from build123d import *

# Parameters (mm, degrees)
SKETCH1_R               = 44.137005248
BOSS_EXTRUDE1_DEPTH     = 2.54
SKETCH2_W               = 7.363975328
SKETCH2_H               = 35.413609254
CUT_EXTRUDE1_DEPTH      = 2.54
BOSS_EXTRUDE2_START     = -6.36773
BOSS_EXTRUDE2_DEPTH     = 35.413609254
CIRPATTERN3_COUNT       = 4
SKETCH6_R               = 46.929171811
SKETCH6_R_2             = 44.137005248
BOSS_EXTRUDE3_DEPTH     = 54.102
CUT_EXTRUDE2_DEPTH      = 86.62546781
CUT_EXTRUDE2_DEPTH_BACK = 86.62546781


with BuildPart() as part:
    # Sketch1 → Boss-Extrude1 (new body)
    with BuildSketch(Plane(origin=(0, 0, 0), x_dir=(1, 0, 0), z_dir=(0, 1, 0))):
        with Locations(Location((0, 0, 0), (0, 0, 270))):
            Circle(SKETCH1_R)
    extrude(amount=BOSS_EXTRUDE1_DEPTH)

    # Sketch2 → Cut-Extrude1 (cut)
    with BuildSketch(Plane(origin=(0, 2.54, 0), x_dir=(1, 0, 0), z_dir=(0, 1, 0))):
        with Locations((0, 24.074534725)):
            Rectangle(SKETCH2_W, SKETCH2_H)
    cut_extrude1 = extrude(amount=-CUT_EXTRUDE1_DEPTH, mode=Mode.SUBTRACT)

    # Sketch3 → Boss-Extrude2 (add)
    with BuildSketch(Plane.XY.offset(BOSS_EXTRUDE2_START)):
        Polygon((3.681987664, 2.54), (-3.464612865, 7.544103563), (2.37831785, 7.544103563), (9.524918378, 2.54), align=None)
    boss_extrude2 = extrude(amount=-BOSS_EXTRUDE2_DEPTH)

    # CirPattern3: Cut-Extrude1, Boss-Extrude2 ×4 about axis
    cirpattern3_axis = Axis((0, 0, 0), (0, 1, 0))
    add([cut_extrude1.rotate(cirpattern3_axis, i * 360 / CIRPATTERN3_COUNT) for i in range(1, CIRPATTERN3_COUNT)], mode=Mode.SUBTRACT)
    add([boss_extrude2.rotate(cirpattern3_axis, i * 360 / CIRPATTERN3_COUNT) for i in range(1, CIRPATTERN3_COUNT)])

    # Sketch6 → Boss-Extrude3 (add)
    with BuildSketch(Plane(origin=(0, 0, 0), x_dir=(1, 0, 0), z_dir=(0, 1, 0))):
        with Locations(Location((0, 0, 0), (0, 0, 270))):
            Circle(SKETCH6_R)
        with Locations(Location((0, 0, 0), (0, 0, 270))):
            Circle(SKETCH6_R_2, mode=Mode.SUBTRACT)
    extrude(amount=BOSS_EXTRUDE3_DEPTH)

    # Sketch7 → Cut-Extrude2 (cut, two sides: drawn at the far end of the back side and taken through both)
    with BuildSketch(Plane(origin=(0, 0, 0), x_dir=(0, 0, -1), z_dir=(1, 0, 0)).offset(-CUT_EXTRUDE2_DEPTH_BACK)):
        Polygon((0, 54.102), (-46.929171811, 5.913652035), (-46.929171811, 54.102), align=None)
    extrude(amount=CUT_EXTRUDE2_DEPTH + CUT_EXTRUDE2_DEPTH_BACK, mode=Mode.SUBTRACT)


solid = part.part
Design review of the part built by this model. Coordinates are the model's own, in mm. A direction names the side the tool comes from. Round coordinates to 2 decimals unless told otherwise and drop trailing zeros. Write each loop counter-clockwise with the first axis right and the second up, starting at its lowest first coordinate (ties: lowest second). Pieces come first, ordered by that corner, then holes. Notation, with made-up numbers: (53.25, 33) -> (110.25, 33) arc R37 ccw to (110.25, 72) -> close; hole circle Ø10 at (44.25, 32). An arc over 180 degrees is marked (long way). One line per item, written item: value. Start each with the question number.
Q1. Add section D-D (y = 49.5). Give the boundary of the cut face in (x, z).
Q2. To check wall thickness, follow probe 1 along X at (y, z) = (40, 0); probe 2 along Y at (x, z) = (-32, -28); probe 3 along X at (y, z) = (27.5, 21). State the ranges of each line that lie inside material, in increasing order.
Q3. Add section C-C (x = 0). Give the boundary of the cut face in (y, z), then the cut area to 3 significant figures.
Q4. Tool access review of faces 1 (the face through (-41.781, 5, -3)), 2 (the face through (0.2, 54.102, -44.4)), 3 (the face through (-0.159, 5.007, 23.827)), 4 (the face through (24, 1, -3.682)): name each direction out of +Z, -Z, +X, -X, +Y, -Y from which nothing blocks a thin tool from reaching the whole face with its end or side.
Q5. The part is to be moulded in two halves that separate along X. For faces 5 (the face through (2.063, 20.661, -46.884)), 6 (the face through (6.368, 5, 3)), 7 (the face through (3.257, 8.703, 44.212)), 8 (the face through (-3.682, 1, 24)), say which applies: pulls with the +X half, pulls with the -X half, needs draft (parallel to the pull), parting line crosses it, or undercut.
Q6. Add section A-A (z = -16.5). Give the boundary of the cut face in (x, y), then the cut area to 3 significant figures.
Q7. Add section B-B (x = 27.5). Give the boundary of the cut face in (y, z), then the cut area to 3 significant figures.
Q8. Insertion check: P1, Ø0.8, axis at x = -1.5, y = 1, coming from the -Z side; P2, Ø3, axis at y = 16, z = -28.5, coming from the -X side; P3, Ø12, axis at y = 46, z = -10, coming from the +X side. Each pin has a flat end and moves straight along its axis. Give the tip position at first contact, or say it passes through.
Response:
1. outline: (-46.71, 4.48) arc R46.93 ccw (long way) to (46.71, 4.48) -> (43.91, 4.48) arc R44.14 cw (long way) to (-43.91, 4.48) -> close
2. probe 1: x = -46.93 to -44.14, 44.14 to 46.93
2. probe 2: y = 0 to 2.54
2. probe 3: x = -41.97 to -38.82, 38.82 to 41.97
3. outline: (0, -46.93) -> (54.1, -46.93) -> (54.1, -44.14) -> (2.54, -44.14) -> (2.54, -41.78) -> (0, -41.78) -> close; (0, -6.37) -> (2.54, -6.37) -> (2.54, 6.37) -> (0, 6.37) -> close; (0, 41.78) -> (2.54, 41.78) -> (2.54, 44.14) -> (8.78, 44.14) -> (5.91, 46.93) -> (0, 46.93) -> close; (5.12, -41.78) -> (7.54, -41.78) -> (7.54, -6.37) -> (5.12, -6.37) -> close; (5.12, 6.37) -> (7.54, 6.37) -> (7.54, 41.78) -> (5.12, 41.78) -> close
3. area: 388 mm^2
4. face 1: +Y
4. face 2: +Z, -Z, +X, -X, +Y
4. face 3: -Y
4. face 4: +Y, -Y
5. face 5: parting line crosses it
5. face 6: undercut
5. face 7: needs draft
5. face 8: undercut
6. outline: (-43.93, 0) -> (-3.68, 0) -> (-3.68, 2.54) -> (-40.94, 2.54) -> (-40.94, 54.1) -> (-43.93, 54.1) -> close; (-3.46, 7.54) -> (3.68, 2.54) -> (3.68, 0) -> (43.93, 0) -> (43.93, 54.1) -> (40.94, 54.1) -> (40.94, 2.54) -> (9.52, 2.54) -> (2.38, 7.54) -> close
6. area: 543 mm^2
7. outline: (0, -38.03) -> (54.1, -38.03) -> (54.1, -34.52) -> (2.54, -34.52) -> (2.54, -3.68) -> (0, -3.68) -> close; (0, 3.68) -> (2.54, 3.68) -> (7.54, -3.46) -> (7.54, 2.38) -> (2.54, 9.52) -> (2.54, 34.52) -> (18.65, 34.52) -> (15.05, 38.03) -> (0, 38.03) -> close
7. area: 435 mm^2
8. P1: stops at z = -46.92
8. P2: stops at x = -38.38
8. P3: stops at x = 46.76
